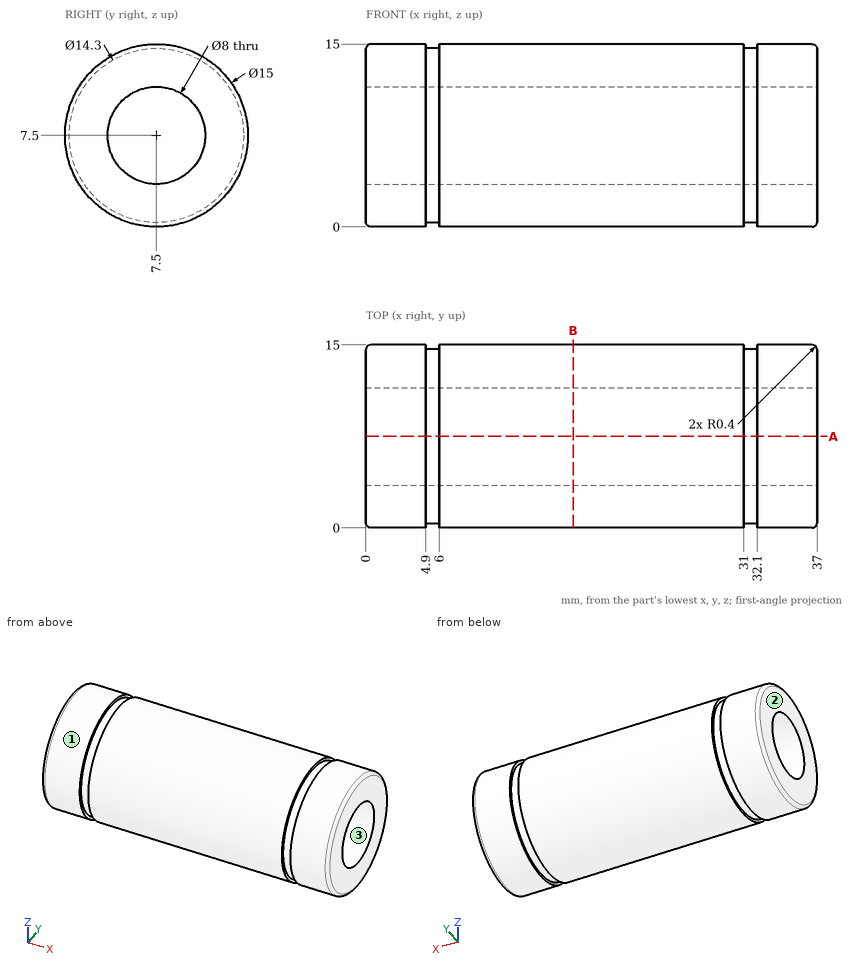
Geometry: see drawing. Coordinates: mm, zero at the bounding-box minimum. Round coordinates to 2 decimals unless told otherwise and drop trailing zeros. Write each loop counter-clockwise with the first axis right and the second up, starting at its lowest first coordinate (ties: lowest second). Pieces come first, ordered by that corner, then holes. Notation, with made-up numbers: M 72,-35 L 86,-35 A20 cw 86,-7 Z; hole C 19.5,2.5 d3. An arc over 180 degrees is marked long. Answer in a Markdown table with one row per item. Add a question column.
(1) Ray query, L1, parallel to Z at x = 18.5, y = 7.5; L2, parallel to X at y = 2.5, z = 12.75; L3, parallel to Y at x = 14, z = 6.75. Return the intervals inside material, ascending.
(2) Cut plane A-A, the plane y = 7.5. Return the cut outline in (x, z).
(3) Cut plane B-B, the plane x = 17. Return the cut outline in (y, z).
(4) Draft query along Y for the marked faces 1, 2 and 3. Return one class per face: pulls with the +Y half, pulls with the -Y half, needs draft (parallel to the pull), parting line crosses it, or undercut.
(5) Contact query for flat-ended pins moving along their axis: pin 1 (4 mm diameter, centred on x = 17.5, z = 13.5, fed in from +Y); pin 2 (4 mm diameter, centred on x = 31, z = 4.5, fed in from +Y); pin 3 (1.5 mm diameter, centred on x = 20, y = 11, fed in from -Z). Output: stop coordinate, or through.
Established:
| question | item | result |
|---|---|---|
| 1 | L1 | 0 to 3.5, 11.5 to 15 |
| 1 | L2 | 0.03 to 4.9, 6 to 31, 32.1 to 36.97 |
| 1 | L3 | 0.04 to 3.57, 11.43 to 14.96 |
| 2 | outline | M 0,0.4 A0.4 ccw 0.4,0 L 4.9,0 L 4.9,0.35 L 6,0.35 L 6,0 L 31,0 L 31,0.35 L 32.1,0.35 L 32.1,0 L 36.6,0 A0.4 ccw 37,0.4 L 37,3.5 L 0,3.5 Z; M 0,11.5 L 37,11.5 L 37,14.6 A0.4 ccw 36.6,15 L 32.1,15 L 32.1,14.65 L 31,14.65 L 31,15 L 6,15 L 6,14.65 L 4.9,14.65 L 4.9,15 L 0.4,15 A0.4 ccw 0,14.6 Z |
| 3 | outline | C 7.5,7.5 d15; hole C 7.5,7.5 d8 |
| 4 | face 1 | parting line crosses it |
| 4 | face 2 | needs draft |
| 4 | face 3 | undercut |
| 5 | pin 1 | y = 13.84 |
| 5 | pin 2 | y = 14.93 |
| 5 | pin 3 | z = 0.52 |
